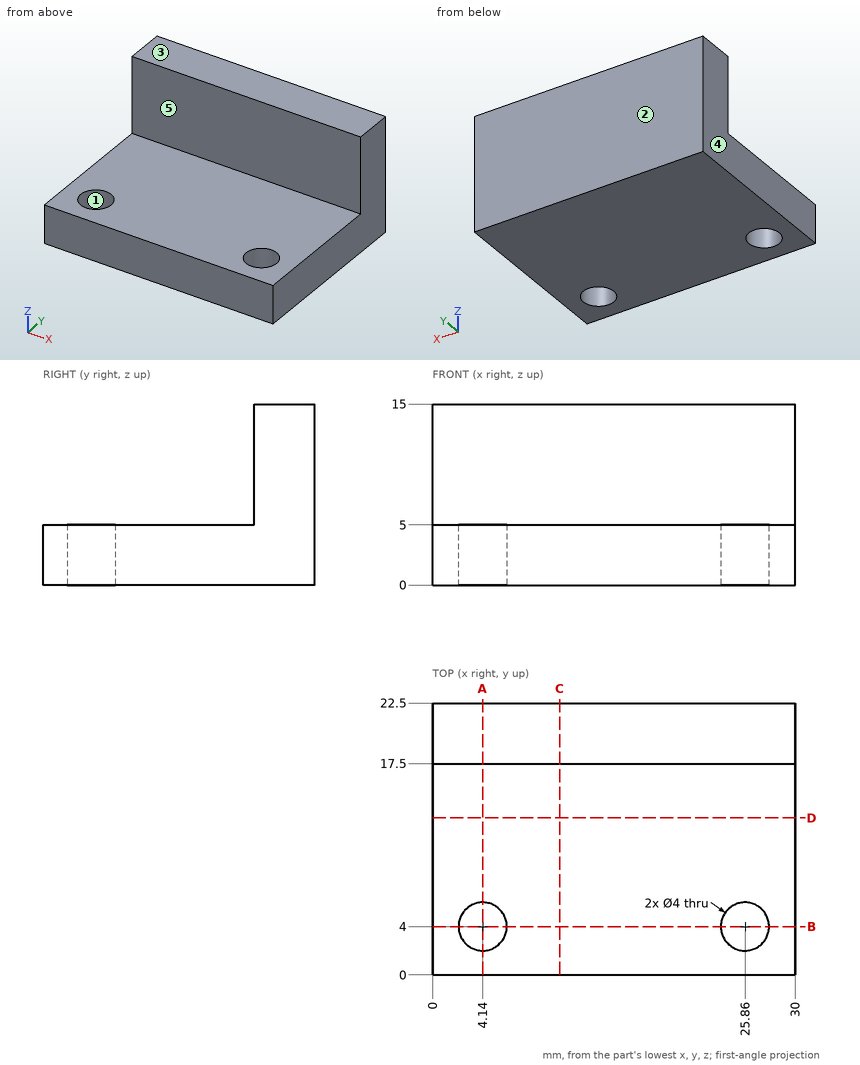
Drawing for the job (mm, zero at the part's lowest x, y, z). A direction names the side the tool comes from. Give positions to 0.01 mm unless a question says otherwise; leave off trailing zeros. Loops run counter-clockwise (first coordinate to the right, second up) from the corner with the lowest first, then second, coordinate; pieces in that order, holes last.
Item 1: Which spindle directions (+Z, -Z, +X, -X, +Y, -Y) get a long thin tool onto all of the face, cutting with end or side? Do the marked faces 4 and 5. Say none if no direction does.
Check values:
face 4: +Z, -Z, -X, +Y, -Y
face 5: +Z, +X, -X, -Y
Item 2: Slice it at B-B (y = 4). Write the cut outline in (x, z).
Check values:
outline: (0, 0) - (2.14, 0) - (2.14, 5) - (0, 5) - close; (6.14, 0) - (23.86, 0) - (23.86, 5) - (6.14, 5) - close; (27.86, 0) - (30, 0) - (30, 5) - (27.86, 5) - close
Item 3: Slice it at D-D (y = 13). Write the cut outline in (x, z), plus the area to 3 significant figures.
Check values:
outline: (0, 0) - (30, 0) - (30, 5) - (0, 5) - close
area: 150 mm2
Item 4: Drop flat-ended pins along their axis: P1, Ø2.5, axis at x = 4.14, y = 4, coming from the +Z side; P2, Ø1.5, axis at x = 8, z = 5, coming from the -Y side; P3, Ø4, axis at x = 19, z = 12.5, coming from the -Y side. Give the stop position or say it passes through.
Check values:
P1: passes through
P2: stops at y = 0
P3: stops at y = 17.5
Item 5: Slice it at A-A (x = 4.14). Write the cut outline in (y, z), plus the area to 4 significant figures.
Check values:
outline: (0, 0) - (2, 0) - (2, 5) - (0, 5) - close; (6, 0) - (22.5, 0) - (22.5, 15) - (17.5, 15) - (17.5, 5) - (6, 5) - close
area: 142.5 mm2
Item 6: Slice it at C-C (x = 10.5). Write the cut outline in (y, z), plus the area to 4 significant figures.
Check values:
outline: (0, 0) - (22.5, 0) - (22.5, 15) - (17.5, 15) - (17.5, 5) - (0, 5) - close
area: 162.5 mm2
Item 7: Drill centre lines: line 1 along Y through (x, z) = (4.14, 1.9); line 2 along Z through (x, y) = (10.5, 1.5); line 3 along Y through (x, z) = (5.25, 13.75). Where is each one in solid material? Low to high.
Check values:
line 1: y = 0 to 2, 6 to 22.5
line 2: z = 0 to 5
line 3: y = 17.5 to 22.5
Item 8: Mould opens along Y. For the marked faces 1, 2 and 3 say: +Y half, -Y half, draft (parallel to the pull), parting line (faces both ways), or undercut.
Check values:
face 1: undercut
face 2: +Y half
face 3: draft
